Input: part model. Units: mm. Frame: model coordinates. Face numbers are marked on the shaded views. A direction names the side the tool comes from. Coordinates: 2 decimals unless noted, no trailing zeros. Order: outer loops, then holes, each group sorted by start corner. A loop starts at its lowest first (then second) coordinate and runs counter-clockwise, first axis right, second up. Notation, with made-up numbers: M 7.25,47.5 L 19.25,47.5 A9 ccw 19.25,52.5 Z; hole C 16.25,36.25 d4. An arc over 180 degrees is marked long. Answer in a Markdown table with one row per item.
from build123d import *

# Parameters (mm, degrees)
F0_R     = 44.45
F1_DEPTH = 120
F2_R     = 50.427629
F3_DEPTH = 30
F4_R     = 9
F5_R     = 10.638423
F6_DEPTH = 150


with BuildPart() as f1:
    # F0 (on Front) → F1 (new body)
    with BuildSketch(Plane.XZ):
        Circle(F0_R)
    extrude(amount=F1_DEPTH)

    # F2 (on Front) → F3 (join)
    with BuildSketch(Plane.XZ):
        Circle(F2_R)
    extrude(amount=-F3_DEPTH)

    # F4
    f4_edges = [f1.edges().sort_by_distance(p)[0] for p in [
        (-50.427629, 30, 0),
    ]]
    fillet(f4_edges, radius=F4_R)

    # F5 (on Front) → F6 (join)
    with BuildSketch(Plane.XZ):
        Circle(F5_R)
    extrude(amount=F6_DEPTH)


solid = f1.part
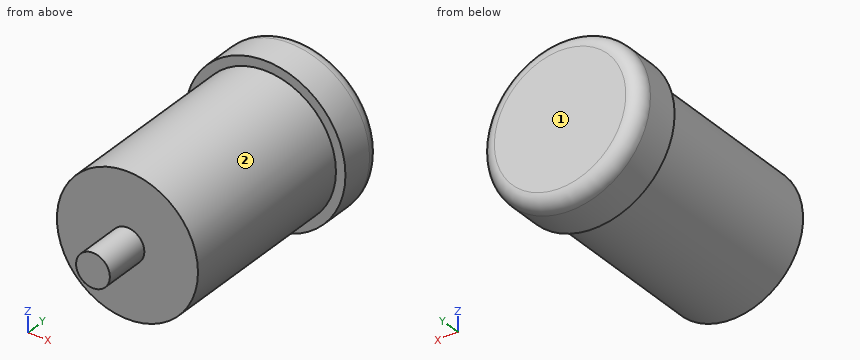
1) Reachability of the marked faces 1 and 2 from +Z, -Z, +X, -X, +Y, -Y: full face, straight path, thin tool, end or side. Return the list, or none.
Resolved:
| item | result |
|---|---|
| face 1 | +Z, -Z, +X, -X, +Y |
| face 2 | -Y |
2) Cut plane C-C, the plane y = -117. Output: boundary loops of the cut face in (x, z).
Resolved:
| item | result |
|---|---|
| outline | C 0,0 d88.9 |
3) Cut plane B-B, the plane x = 0. Output: boundary loops of the cut face in (y, z), and give its area (3 significant figures).
Resolved:
| item | result |
|---|---|
| outline | M -150,-10.64 L -120,-10.64 L -120,-44.45 L 0,-44.45 L 0,-50.43 L 21,-50.43 A9 ccw 30,-41.43 L 30,41.43 A9 ccw 21,50.43 L 0,50.43 L 0,44.45 L -120,44.45 L -120,10.64 L -150,10.64 Z |
| area | 14,300 mm2 |
4) Material intervals for probe 1 along Y at (x, z) = (-18, -1); probe 2 along Z at (x, y) = (-16, -14.5); probe 3 along X at (y, z) = (-7, 2), sorted ascending.
Resolved:
| item | result |
|---|---|
| probe 1 | y = -120 to 30 |
| probe 2 | z = -41.47 to 41.47 |
| probe 3 | x = -44.4 to 44.4 |
5) Contact query for flat-ended pins moving along their axis: pin 1 (6 mm diameter, centred on y = -21.5, z = -24, fed in from -X); pin 2 (12 mm diameter, centred on y = 0.5, z = -16, fed in from +X); pin 3 (6 mm diameter, centred on y = -123.5, z = -11.5, fed in from -X). Output: stop coordinate, or through.
Resolved:
| item | result |
|---|---|
| pin 1 | stops at x = -39.18 |
| pin 2 | stops at x = 49.43 |
| pin 3 | stops at x = -6.4 |
6) Cut plane A-A, the plane z = 0. Output: boundary loops of the cut face in (x, y).
Resolved:
| item | result |
|---|---|
| outline | M -50.43,0 L -44.45,0 L -44.45,-120 L -10.64,-120 L -10.64,-150 L 10.64,-150 L 10.64,-120 L 44.45,-120 L 44.45,0 L 50.43,0 L 50.43,21 A9 ccw 41.43,30 L -41.43,30 A9 ccw -50.43,21 Z |
